The listing builds one solid part. Answer for the finished solid, in the listing's coordinates (mm). Round coordinates to 2 decimals unless told otherwise and drop trailing zeros. Loops run counter-clockwise (first coordinate to the right, second up) from the corner with the lowest first, then second, coordinate; pieces in that order, holes last. Notation, with made-up numbers: (44.25, -28) -> (52.25, -28) arc R19 cw to (52.25, -17) -> close; hole circle Ø1 at (75.5, 58.5). An arc over 180 degrees is marked (long way). Write each question's results on one line, items separated by ' | '. Start each with the question number.
(1) Straight lines are drawn through the part: probe 1 along Z at (x, y) = (-0.05, 3); probe 2 along Z at (x, y) = (-0.7, 2); probe 3 along Y at (x, z) = (-1.6, 0.65). For each, find the intervals that lie inside material, in ascending order.
(2) The part is cut by section A-A (y = -10). Determine the outline of the cut face in (x, z), plus the area to 3 significant figures.
(3) A flat-ended cylindrical pin translates along its axis: pin 1 (0.6 mm diameter, centred on x = 0, z = -0.5, fed in from -Y). Find the tip coordinate at first contact, or state that the pin passes through.
(4) The part is cut by section B-B (y = 3). Determine the outline of the cut face in (x, z), plus the area to 3 significant figures.
```python
from build123d import *

# Parameters (mm, degrees)
CUT_EXTRUDE1_DEPTH  = 1
SKETCH3_R           = 0.25
BOSS_EXTRUDE1_DEPTH = 24.5
SKETCH4_R           = 0.25
BOSS_EXTRUDE2_DEPTH = 1.2
SKETCH5_R           = 0.25
BOSS_EXTRUDE3_DEPTH = 2


with BuildPart() as part:
    # Sketch1 → Revolve1 (revolve)
    with BuildSketch(Plane.XY):
        with BuildLine():
            Line((0, 0), (0, 8.75))
            Line((0, 8.75), (0.1, 8.75))
            ThreePointArc((0.1, 8.75), (1.797056275, 8.047056275), (2.5, 6.35))
            Line((2.5, 6.35), (2.5, 1))
            Line((2.5, 1), (2.85, 1))
            Line((2.85, 1), (2.85, 0))
            Line((2.85, 0), (0, 0))
        make_face()
    revolve(axis=Axis((0, 0, 0), (0, 1, 0)))

    # Sketch2 → Cut-Extrude1 (cut)
    with BuildSketch(Plane.XZ):
        with BuildLine():
            Line((-1.167261753, 2.6), (1.167261753, 2.6))
            ThreePointArc((1.167261753, 2.6), (0, 2.85), (-1.167261753, 2.6))
        make_face()
    extrude(amount=-CUT_EXTRUDE1_DEPTH, mode=Mode.SUBTRACT)

    # Sketch3 → Boss-Extrude1 (add)
    with BuildSketch(Plane.XZ):
        with Locations((0, -2.15)):
            Circle(SKETCH3_R)
        with Locations((0, 2.15)):
            Circle(SKETCH3_R)
        with Locations((0, -0.716666667)):
            Circle(SKETCH3_R)
        with Locations((0, 0.716666667)):
            Circle(SKETCH3_R)
    extrude(amount=BOSS_EXTRUDE1_DEPTH)

    # Sketch4 → Boss-Extrude2 (add)
    with BuildSketch(Plane.XZ.offset(24.5)):
        with Locations((0, 2.15)):
            Circle(SKETCH4_R)
        with Locations((0, -0.716666667)):
            Circle(SKETCH4_R)
    extrude(amount=BOSS_EXTRUDE2_DEPTH)

    # Sketch5 → Boss-Extrude3 (add)
    with BuildSketch(Plane.XZ.offset(24.5)):
        with Locations((0, 0.716666667)):
            Circle(SKETCH5_R)
    extrude(amount=BOSS_EXTRUDE3_DEPTH)


solid = part.part
```
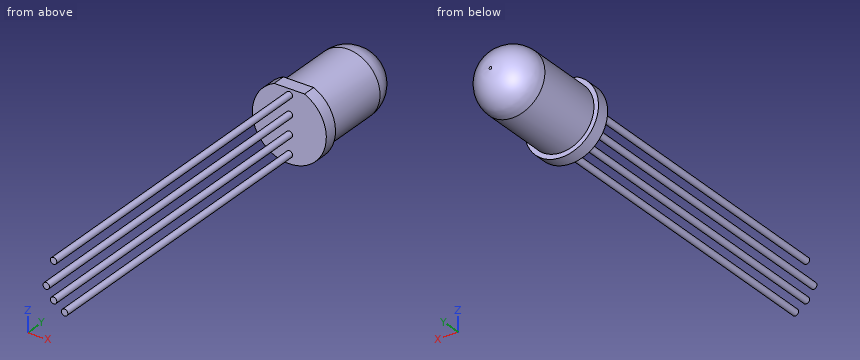
Checked values:
1) probe 1: z = -2.5 to 2.5 | probe 2: z = -2.4 to 2.4 | probe 3: y = 0 to 8.11
2) outline: circle Ø0.5 at (0, -2.15); circle Ø0.5 at (0, -0.72); circle Ø0.5 at (0, 0.72); circle Ø0.5 at (0, 2.15) | area: 0.785 mm2
3) pin 1: stops at y = -25.7
4) outline: circle Ø5 at (0, 0) | area: 19.6 mm2
